```python
from build123d import *

# Parameters (mm, degrees)
SKETCH024_R = 4
PAD_DEPTH   = 5.5


with BuildPart() as part:
    # Sketch024 → Pad (new body)
    with BuildSketch(Plane.XY):
        Polygon((7.5055534995, 0), (3.7527767497, 6.5), (-3.7527767497, 6.5), (-7.5055534995, 0), (-3.7527767497, -6.5), (3.7527767497, -6.5), align=None)
        Circle(SKETCH024_R, mode=Mode.SUBTRACT)
    extrude(amount=PAD_DEPTH)

    # Sketch025 → Revolution005 (revolve)
    with BuildSketch(Plane.XZ):
        with BuildLine():
            Line((4, 5.5), (5.85, 5.5))
            Line((5.85, 5.5), (5.85, 7.4))
            ThreePointArc((5.85, 7.4), (5.7035533906, 7.7535533906), (5.35, 7.9))
            Line((5.35, 7.9), (4, 7.9))
            Line((4, 7.9), (4, 5.5))
        make_face()
    revolve(axis=Axis((0, 0, 0), (0, 0, 1)))

    # Sketch026 → Groove (revolve, cut)
    with BuildSketch(Plane.XZ):
        Polygon((7.5055534995, 5.5), (6.5055534995, 5.5), (7.5055534995, 5), align=None)
        Polygon((7.5055534995, 0), (6.5055534995, 0), (7.5055534995, 0.5), align=None)
    revolve(axis=Axis((0, 0, 0), (0, 0, 1)), mode=Mode.SUBTRACT)


solid = part.part
```
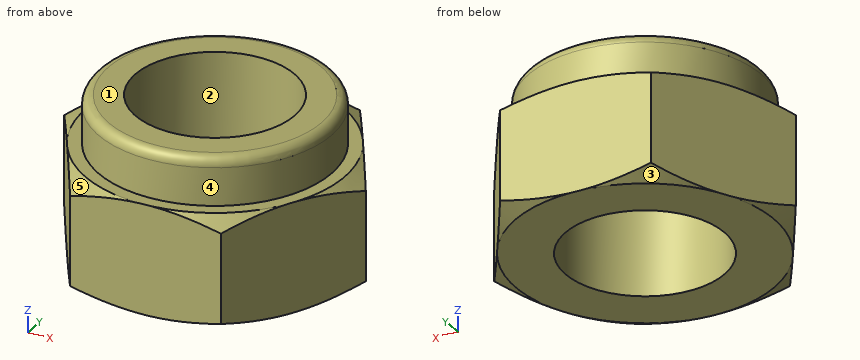
CAD build for the part. Positions are in the model's coordinates, mm. Face numbers are marked on the shaded views. A direction names the side the tool comes from. Round coordinates to 2 decimals unless told otherwise and drop trailing zeros. Order: outer loops, then holes, each group sorted by start corner. A loop starts at its lowest first (then second) coordinate and runs counter-clockwise, first axis right, second up. Notation, with made-up numbers: (-38.5, 60.5) - (-21.5, 60.5) arc R6 ccw to (-21.5, 66.5) - close; hole circle Ø4 at (28.25, 11). An arc over 180 degrees is marked (long way). Answer in a Markdown table with one row per item. Add a question column.
(1) Mould opens along Y. For the marked faces 1, 2 and 3 say: +Y half, -Y half, draft (parallel to the pull), parting line (faces both ways), or undercut.
(2) Band-saw the part on C-C on z = 6. List the corners of the cut face in (x, y), and give its area (3 significant figures).
(3) 3-axis set-ups, long thin cutter, end or side, ignore diameter. For the marked faces 4 and 5: which of +Z, -Z, +X, -X, +Y, -Y reach the whole face in a straight line?
(4) Band-saw the part on B-B on x = 0. List the corners of the cut face in (y, z), and give its area (3 significant figures).
(5) Drop a flat-ended pin along its axis: pin 1 Ø1.5 at (y, z) = (-0.5, 3) entering from -X. Give the stop position or say it passes through.
(6) Band-saw the part on A-A on z = 2. List the corners of the cut face in (x, y).
(7) Probe L1, parallel to Y at x = 0, z = 5.75; L2, parallel to Y at x = 0, z = 2; L3, parallel to Z at x = 2, y = 5. List the from-to ranges inside material, lowest first. Write a range as [from, to].
Data:
| question | item | result |
|---|---|---|
| 1 | face 1 | draft |
| 1 | face 2 | undercut |
| 1 | face 3 | +Y half |
| 2 | outline | circle Ø11.7 at (0, 0); hole circle Ø8 at (0, 0) |
| 2 | area | 57.2 mm^2 |
| 3 | face 4 | +Z |
| 3 | face 5 | +Z, -X, -Y |
| 4 | outline | (-6.5, 0) - (-4, 0) - (-4, 7.9) - (-5.35, 7.9) arc R0.5 ccw to (-5.85, 7.4) - (-5.85, 5.5) - (-6.5, 5.5) - close; (4, 0) - (6.5, 0) - (6.5, 5.5) - (5.85, 5.5) - (5.85, 7.4) arc R0.5 ccw to (5.35, 7.9) - (4, 7.9) - close |
| 4 | area | 36.3 mm^2 |
| 5 | pin 1 | stops at x = -7.51 |
| 6 | outline | (-7.51, 0) - (-3.75, -6.5) - (3.75, -6.5) - (7.51, 0) - (3.75, 6.5) - (-3.75, 6.5) - close; hole circle Ø8 at (0, 0) |
| 7 | L1 | y = [-5.85, -4], [4, 5.85] |
| 7 | L2 | y = [-6.5, -4], [4, 6.5] |
| 7 | L3 | z = [0, 7.9] |
